Autodesk Inventor part; units mm, degrees
ref_plane "YZ Plane" through (0, 0, 0) normal (1, 0, 0) x (0, 1, 0)
ref_plane "XZ Plane" through (0, 0, 0) normal (0, 1, 0) x (-1, 0, 0)
ref_plane "XY Plane" through (0, 0, 0) normal (0, 0, 1) x (1, 0, 0)
sketch "Sketch1" plane through (0, 0, 0) normal (0, 1, 0) x (-1, 0, 0)
  line L0 (65, 0) -> (65, -100)
  line L1 (65, -100) -> (0, -100)
  line L2 (0, -100) -> (0, 0)
  line L3 (8, -34) -> (57, -34) construction
  line L4 (57, -34) -> (57, -92) construction
  line L5 (57, -92) -> (8, -92) construction
  line L6 (8, -92) -> (8, -34) construction
  circle A0 centre (57, -34) radius 1.35
  circle A1 centre (57, -92) radius 1.35
  circle A2 centre (8, -34) radius 1.35
  circle A3 centre (8, -92) radius 1.35
  line L7 (49, -42) -> (16, -42)
  line L8 (16, -42) -> (16, -84)
  line L9 (16, -84) -> (49, -84)
  line L10 (49, -84) -> (49, -42)
  line L11 (49, 0) -> (16, 0) construction
  line L12 (16, 0) -> (16, -26)
  line L13 (16, -26) -> (49, -26)
  line L14 (49, -26) -> (49, 0)
  line L15 (0, 0) -> (16, 0)
  line L16 (49, 0) -> (65, 0)
  point P0 (32.5, -34)
  dimension "d0" = 49
  dimension "d1" = 58
  dimension "d2" = 2.7
  dimension "d3" = 100
  dimension "d4" = 65
  dimension "d5" = 8
  dimension "d7" = 8
  dimension "d8" = 8
  dimension "d9" = 8
  dimension "d10" = 8
  dimension "d11" = 8
  dimension "d15" = 8
extrude "Extrusion1" add sketch "Sketch1" along normal blind 2
fillet "Fillet1" radius 2 12 edges at (-49, 1, -84) (-49, 1, -42) (-16, 1, -42) (-16, 1, -84) (-65, 1, -100) (0, 1, -100) (0, 1, 0) (-65, 1, 0) (-49, 1, 0) (-49, 1, -26) (-16, 1, -26) (-16, 1, 0)
equation "\"d5\" = -0.5 * d0 + 0.5 * d4"
equation "\"d7\" = d5"
equation "\"d8\" = d5"
equation "\"d9\" = d5"
equation "\"d10\" = d5"
equation "\"d11\" = d5"
equation "\"d15\" = d5"
properties part number "targetpart"
Verification items for the finished model (mm, model axes). A direction names the side the tool comes from. Round coordinates to 2 decimals unless told otherwise and drop trailing zeros. Loops run counter-clockwise (first coordinate to the right, second up) from the corner with the lowest first, then second, coordinate; pieces in that order, holes last. Notation, with made-up numbers: (-1.5, 26) - (3.5, 26) arc R29 ccw to (3.5, 64) - close; hole circle Ø8 at (5.5, 84.25). An arc over 180 degrees is marked (long way). Use a Markdown table: item, result. Add a question column.
1. Section check A-A, the plane z = -10.5. Record the boundary of the cut face in (x, y), plus the area to 3 significant figures.
2. Section check D-D, the plane x = -26. Record the boundary of the cut face in (y, z), plus the area to 3 significant figures.
3. Thickness scan on probe 1 along X at (y, z) = (1.5, -92); probe 2 along Z at (x, y) = (-57, 1.95); probe 3 along X at (y, z) = (1.75, -51.5). Record the ranges inside material, lowest first. Write a range as [from, to].
4. Release check for a two-part mould opening along X. For faces 4 (the face through (-48.4, 1.01, -83.43)), 5 (the face through (-0.6, 1.01, -0.57)), 6 (the face through (-65, 1, -49)), 7 (the face through (-49, 1, -63)) record: released by +X, released by -X, zero draft, split by the parting line, or undercut.
5. Access from +Z, -Z, +X, -X, +Y, -Y to the whole of each face (thin tool, end or side, straight path). Record for faces 1 (the face through (-49.6, 1.01, -0.57)), 2 (the face through (-8, 1, 0)), 3 (the face through (-16, 1, -63)).
6. Gauge pin test, flat end, axial feed: pin 1 (1.6 mm diameter, centred on x = -8, z = -34, fed in from -Y). Record the tip position at first contact, or that the pin passes through.
7. Section check C-C, the plane y = 0.75. Record the boundary of the cut face in (x, z), plus the area to 3 significant figures.
8. Section check B-B, the plane x = -8. Record the boundary of the cut face in (y, z), plus the area to 3 significant figures.
Checks:
| question | item | result |
|---|---|---|
| 1 | outline | (-65, 0) - (-49, 0) - (-49, 2) - (-65, 2) - close; (-16, 0) - (0, 0) - (0, 2) - (-16, 2) - close |
| 1 | area | 64.0 mm^2 |
| 2 | outline | (0, -100) - (2, -100) - (2, -84) - (0, -84) - close; (0, -42) - (2, -42) - (2, -26) - (0, -26) - close |
| 2 | area | 64.0 mm^2 |
| 3 | probe 1 | x = [-65, -58.35], [-55.65, -9.35], [-6.65, 0] |
| 3 | probe 2 | z = [-100, -93.35], [-90.65, -35.35], [-32.65, 0] |
| 3 | probe 3 | x = [-65, -49], [-16, 0] |
| 4 | face 4 | undercut |
| 4 | face 5 | released by +X |
| 4 | face 6 | released by -X |
| 4 | face 7 | undercut |
| 5 | face 1 | +Z, +Y, -Y |
| 5 | face 2 | +Z, +X, -X, +Y, -Y |
| 5 | face 3 | +Y, -Y |
| 6 | pin 1 | passes through |
| 7 | outline | (-65, -98) arc R2 ccw to (-63, -100) - (-2, -100) arc R2 ccw to (0, -98) - (0, -2) arc R2 ccw to (-2, 0) - (-14, 0) arc R2 ccw to (-16, -2) - (-16, -24) arc R2 cw to (-18, -26) - (-47, -26) arc R2 cw to (-49, -24) - (-49, -2) arc R2 ccw to (-51, 0) - (-63, 0) arc R2 ccw to (-65, -2) - close; hole circle Ø2.7 at (-57, -92); hole circle Ø2.7 at (-57, -34); hole (-49, -82) arc R2 ccw to (-47, -84) - (-18, -84) arc R2 ccw to (-16, -82) - (-16, -44) arc R2 ccw to (-18, -42) - (-47, -42) arc R2 ccw to (-49, -44) - close; hole circle Ø2.7 at (-8, -92); hole circle Ø2.7 at (-8, -34) |
| 7 | area | 4,230 mm^2 |
| 8 | outline | (0, -100) - (2, -100) - (2, -93.35) - (0, -93.35) - close; (0, -90.65) - (2, -90.65) - (2, -35.35) - (0, -35.35) - close; (0, -32.65) - (2, -32.65) - (2, 0) - (0, 0) - close |
| 8 | area | 189 mm^2 |
